```python
from build123d import *

# Parameters (mm, degrees)
BOSS_EXTRUDE1_DEPTH = 1.5875
SKETCH2_R           = 2.1
CUT_EXTRUDE1_DEPTH  = 243.144751389
SKETCH3_W           = 86
SKETCH3_H           = 86
SKETCH3_R           = 1.65
BOSS_EXTRUDE2_DEPTH = 3.175
FILLET1_R           = 4
SKETCH5_R           = 2.1
CUT_EXTRUDE3_DEPTH  = 244.842327386
SKETCH6_R           = 21.1
BOSS_EXTRUDE3_DEPTH = 3.175
FILLET2_R           = 4


with BuildPart() as part:
    # Sketch1 → Boss-Extrude1 (new, symmetric)
    with BuildSketch(Plane.YZ):
        with BuildLine():
            Line((-208, 32), (208, 32))
            ThreePointArc((208, 32), (240, 0), (208, -32))
            Line((208, -32), (-208, -32))
            ThreePointArc((-208, -32), (-240, 0), (-208, 32))
        make_face()
    extrude(amount=BOSS_EXTRUDE1_DEPTH, both=True)

    # Sketch2 → Cut-Extrude1 (cut, through all)
    with BuildSketch(Plane.YZ.offset(1.5875)):
        with Locations(Location((-208, 12, 0), (0, 0, 270))):
            Circle(SKETCH2_R)
        with Locations(Location((-197.607695155, 6, 0), (0, 0, 270))):
            Circle(SKETCH2_R)
        with Locations(Location((-197.607695155, -6, 0), (0, 0, 270))):
            Circle(SKETCH2_R)
        with Locations(Location((-208, -12, 0), (0, 0, 270))):
            Circle(SKETCH2_R)
        with Locations(Location((-218.392304845, -6, 0), (0, 0, 270))):
            Circle(SKETCH2_R)
        with Locations(Location((-218.392304845, 6, 0), (0, 0, 270))):
            Circle(SKETCH2_R)
    extrude(amount=-CUT_EXTRUDE1_DEPTH, mode=Mode.SUBTRACT)

    # Sketch3 → Boss-Extrude2 (add)
    with BuildSketch(Plane.YZ.offset(1.5875)):
        with Locations((-112, 0)):
            Rectangle(SKETCH3_W, SKETCH3_H)
        with Locations(Location((-146, 34, 0), (0, 0, 270))):
            Circle(SKETCH3_R, mode=Mode.SUBTRACT)
        with Locations(Location((-78, 34, 0), (0, 0, 270))):
            Circle(SKETCH3_R, mode=Mode.SUBTRACT)
        with Locations(Location((-78, -34, 0), (0, 0, 270))):
            Circle(SKETCH3_R, mode=Mode.SUBTRACT)
        with Locations(Location((-146, -34, 0), (0, 0, 270))):
            Circle(SKETCH3_R, mode=Mode.SUBTRACT)
    extrude(amount=-BOSS_EXTRUDE2_DEPTH)

    # Fillet1
    fillet1_edges = [part.edges().sort_by_distance(p)[0] for p in [
        (0, -69, 32),
        (0, -155, 32),
        (0, -155, -32),
        (0, -155, -43),
        (0, -69, 43),
        (0, -69, -32),
        (0, -155, 43),
        (0, -69, -43),
    ]]
    fillet(fillet1_edges, radius=FILLET1_R)

    # Sketch5 → Cut-Extrude3 (cut, through all)
    with BuildSketch(Plane.YZ.offset(1.5875)):
        with Locations(Location((-208, 28, 0), (0, 0, 270))):
            Circle(SKETCH5_R)
        with Locations(Location((-176, 28, 0), (0, 0, 270))):
            Circle(SKETCH5_R)
        with Locations(Location((-48, 28, 0), (0, 0, 270))):
            Circle(SKETCH5_R)
        with Locations(Location((-16, 28, 0), (0, 0, 270))):
            Circle(SKETCH5_R)
        with Locations(Location((16, 28, 0), (0, 0, 270))):
            Circle(SKETCH5_R)
        with Locations(Location((48, 28, 0), (0, 0, 270))):
            Circle(SKETCH5_R)
        with Locations(Location((80, 28, 0), (0, 0, 270))):
            Circle(SKETCH5_R)
        with Locations(Location((112, 28, 0), (0, 0, 270))):
            Circle(SKETCH5_R)
        with Locations(Location((144, 28, 0), (0, 0, 270))):
            Circle(SKETCH5_R)
        with Locations(Location((176, 28, 0), (0, 0, 270))):
            Circle(SKETCH5_R)
        with Locations(Location((176, -28, 0), (0, 0, 90))):
            Circle(SKETCH5_R)
        with Locations(Location((144, -28, 0), (0, 0, 90))):
            Circle(SKETCH5_R)
        with Locations(Location((112, -28, 0), (0, 0, 90))):
            Circle(SKETCH5_R)
        with Locations(Location((80, -28, 0), (0, 0, 90))):
            Circle(SKETCH5_R)
        with Locations(Location((48, -28, 0), (0, 0, 90))):
            Circle(SKETCH5_R)
        with Locations(Location((16, -28, 0), (0, 0, 90))):
            Circle(SKETCH5_R)
        with Locations(Location((-16, -28, 0), (0, 0, 90))):
            Circle(SKETCH5_R)
        with Locations(Location((-48, -28, 0), (0, 0, 90))):
            Circle(SKETCH5_R)
        with Locations(Location((-176, -28, 0), (0, 0, 90))):
            Circle(SKETCH5_R)
        with Locations(Location((-208, -28, 0), (0, 0, 90))):
            Circle(SKETCH5_R)
        with Locations(Location((208, 28, 0), (0, 0, 270))):
            Circle(SKETCH5_R)
        with Locations(Location((208, -28, 0), (0, 0, 90))):
            Circle(SKETCH5_R)
    extrude(amount=-CUT_EXTRUDE3_DEPTH, mode=Mode.SUBTRACT)

    # Sketch6 → Boss-Extrude3 (add)
    with BuildSketch(Plane.YZ.offset(1.5875)):
        with BuildLine():
            ThreePointArc((208, 32), (230.627416998, 22.627416998), (240, 0))
            Line((240, 0), (240, 107))
            Line((240, 107), (176, 107))
            Line((176, 107), (176, 32))
            Line((176, 32), (208, 32))
        make_face()
        with Locations(Location((208, 75, 0), (0, 0, 270))):
            Circle(SKETCH6_R, mode=Mode.SUBTRACT)
    extrude(amount=-BOSS_EXTRUDE3_DEPTH)

    # Fillet2
    fillet2_edges = [part.edges().sort_by_distance(p)[0] for p in [
        (0, 240, 107),
        (0, 176, 107),
        (0, 176, 32),
    ]]
    fillet(fillet2_edges, radius=FILLET2_R)


solid = part.part
```
Input: part model. Units: mm. Frame: model coordinates. Round coordinates to 2 decimals unless told otherwise and drop trailing zeros. Loops run counter-clockwise (first coordinate to the right, second up) from the corner with the lowest first, then second, coordinate; pieces in that order, holes last. Notation, with made-up numbers: (-5, -17.5) - (44, -17.5) arc R27 cw to (44, 0.5) - close; hole circle Ø2 at (43, 2). An arc over 180 degrees is marked (long way). One line per item, written item: value. Start each with the question number.
(1) Draft query along Z for faces 1 (the flat face through (-1.588, -3, 0)), 2 (the cylindrical face through (0.02, 187.4, 79.57)), 3 (the cylindrical face through (0.022, -239.992, -0.704)). Return one class per face: +Z half, -Z half, draft (parallel to the pull), parting line (faces both ways), or undercut.
(2) Section A-A, the plane y = 103. Return loops of the section in (x, z).
(3) Contact query for a flat-ended pin moving along its axis: P1, Ø1, axis at x = 0, z = 3, coming from the -Y side. Output: stop coordinate, or through.
(4) Section B-B, the plane x = -0.25. Count the separate pieces of the cut face and the enclosed holes in it, plus the area to 3 significant figures.
(5) Section C-C, the plane z = -21.5. Return loops of the section in (x, y).
(6) Ray query, line 1 (Z direction, x = 0.45, y = 144); line 2 (Z direction, x = 0.05, y = -208); line 3 (Y direction, x = 1.1, z = 75.5). Return the intervals inside material, ascending. Write a range as [from, to].
Results below:
1. face 1: draft
1. face 2: undercut
1. face 3: parting line
2. outline: (-1.59, -32) - (1.59, -32) - (1.59, 32) - (-1.59, 32) - close
3. P1: y = -239.9
4. separate pieces: 1
4. enclosed holes: 33
4. area: 34,900 mm^2
5. outline: (-1.59, -231.7) - (1.59, -231.7) - (1.59, 231.7) - (-1.59, 231.7) - close
6. line 1: [-32, -30.1], [-25.9, 25.9], [30.1, 32]
6. line 2: [-32, -30.1], [-25.9, -14.1], [-9.9, 9.9], [14.1, 25.9], [30.1, 32]
6. line 3: [176, 186.91], [229.09, 240]
